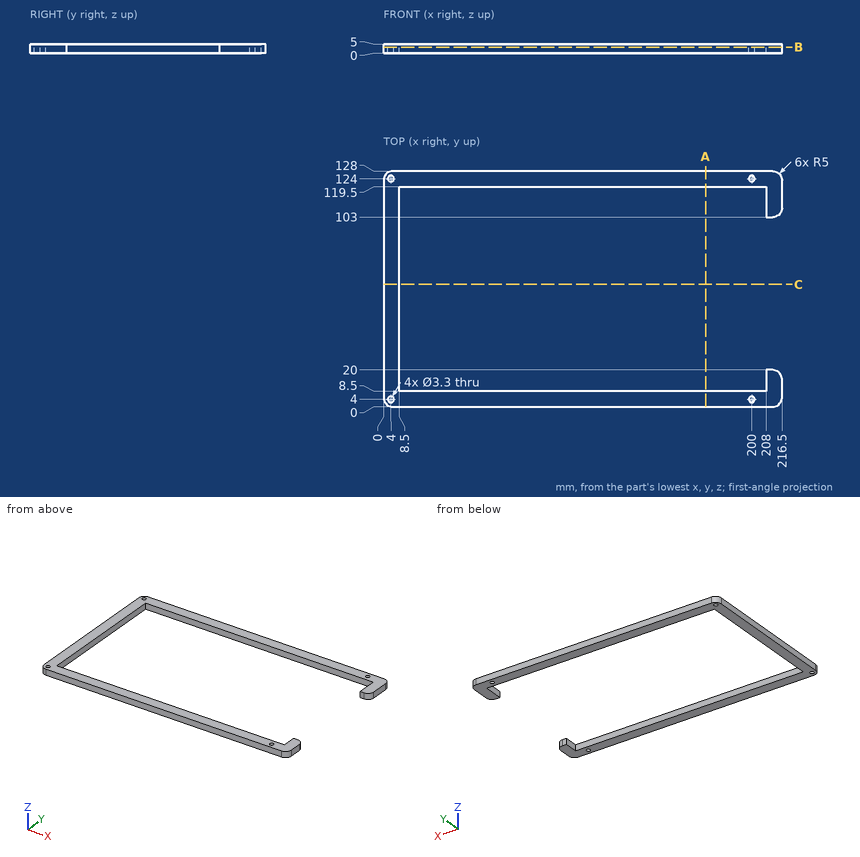
Geometry: see drawing. Coordinates: mm, zero at the bounding-box minimum. Coordinates: 2 decimals unless noted, no trailing zeros. Write each loop counter-clockwise with the first axis right and the second up, starting at its lowest first coordinate (ties: lowest second). Pieces come first, ordered by that corner, then holes.
1) Section C-C on y = 66.5. Output: boundary loops of the cut face in (x, z).
2) Section A-A on x = 175. Output: boundary loops of the cut face in (y, z).
3) Pin query (flat end, axial travel): pin 1 Ø1.5 at (y, z) = (50.5, 1.5) entering from +X. Return the tip coordinate at first contact, or that it passes through.
4) Material intervals for line 1 along Y through (x, z) = (175, 4.05); line 2 along X through (y, z) = (4, 2.75); line 3 along X through (y, z) = (112, 2.1), sorted ascending.
5) Section B-B on z = 3.35. Output: boundary loops of the cut face in (x, y).
Check result:
1. outline: (0, 0) - (8.5, 0) - (8.5, 5) - (0, 5) - close
2. outline: (0, 0) - (8.5, 0) - (8.5, 5) - (0, 5) - close; (119.5, 0) - (128, 0) - (128, 5) - (119.5, 5) - close
3. pin 1: stops at x = 8.5
4. line 1: y = 0 to 8.5, 119.5 to 128
4. line 2: x = 0.1 to 2.35, 5.65 to 198.35, 201.65 to 216.4
4. line 3: x = 0 to 8.5, 208 to 216.5
5. outline: (0, 5) arc R5 ccw to (5, 0) - (211.5, 0) arc R5 ccw to (216.5, 5) - (216.5, 15) arc R5 ccw to (211.5, 20) - (208, 20) - (208, 8.5) - (8.5, 8.5) - (8.5, 119.5) - (208, 119.5) - (208, 103) - (211.5, 103) arc R5 ccw to (216.5, 108) - (216.5, 123) arc R5 ccw to (211.5, 128) - (5, 128) arc R5 ccw to (0, 123) - close; hole circle Ø3.3 at (4, 4); hole circle Ø3.3 at (4, 124); hole circle Ø3.3 at (200, 4); hole circle Ø3.3 at (200, 124)
